```python
from build123d import *

# Parameters (mm, degrees)
SKETCH1_W           = 24
SKETCH1_H           = 24
BOSS_EXTRUDE1_DEPTH = 6
SKETCH2_W           = 24
SKETCH2_H           = 6
BOSS_EXTRUDE2_DEPTH = 30
SKETCH3_W           = 24
SKETCH3_H           = 6
BOSS_EXTRUDE3_DEPTH = 6
SKETCH4_W           = 24
SKETCH4_H           = 6
BOSS_EXTRUDE4_DEPTH = 6
SKETCH5_W           = 10
SKETCH5_H           = 6
BOSS_EXTRUDE5_DEPTH = 8
FILLET1_R           = 5
FILLET2_R           = 2
FILLET3_R           = 2
SKETCH6_W           = 10
SKETCH6_H           = 6
BOSS_EXTRUDE6_DEPTH = 8
FILLET4_R           = 5
FILLET5_R           = 2
SKETCH7_R           = 1.775
CUT_EXTRUDE1_DEPTH  = 42.568724431
CUT_EXTRUDE2_REACH  = 51.934
SKETCH8_R           = 1.75


with BuildPart() as part:
    # Sketch1 → Boss-Extrude1 (new body)
    with BuildSketch(Plane(origin=(0, 0, 0), x_dir=(1, 0, 0), z_dir=(0, 1, 0))):
        with Locations((1.896724894, -0.667948192)):
            Rectangle(SKETCH1_W, SKETCH1_H)
    extrude(amount=BOSS_EXTRUDE1_DEPTH)

    # Sketch2 → Boss-Extrude2 (add)
    with BuildSketch(Plane(origin=(0, 6, 0), x_dir=(1, 0, 0), z_dir=(0, 1, 0))):
        with Locations((1.896724894, -6.462948192)):
            Rectangle(SKETCH2_W, SKETCH2_H)
        with Locations((1.896724894, 5.127051808)):
            Rectangle(SKETCH2_W, SKETCH2_H)
    extrude(amount=BOSS_EXTRUDE2_DEPTH)

    # Sketch3 → Boss-Extrude3 (add)
    with BuildSketch(Plane.XY.offset(12.667948192)):
        with Locations((1.896724894, 3)):
            Rectangle(SKETCH3_W, SKETCH3_H)
    extrude(amount=BOSS_EXTRUDE3_DEPTH)

    # Sketch4 → Boss-Extrude4 (add)
    with BuildSketch(Plane(origin=(0, 0, -11.332051808), x_dir=(-1, 0, 0), z_dir=(0, 0, -1))):
        with Locations((-1.896724894, 3)):
            Rectangle(SKETCH4_W, SKETCH4_H)
    extrude(amount=BOSS_EXTRUDE4_DEPTH)

    # Sketch5 → Boss-Extrude5 (add)
    with BuildSketch(Plane(origin=(13.896724894, 0, 0), x_dir=(0, 0, -1), z_dir=(1, 0, 0))):
        with Locations((-0.667948192, 3)):
            Rectangle(SKETCH5_W, SKETCH5_H)
    extrude(amount=BOSS_EXTRUDE5_DEPTH)

    # Fillet1
    # the kernel refuses this fillet: 5 mm, written as the material it adds along each edge
    with BuildSketch(Plane(origin=(13.896724894, 0, -4.332051808), x_dir=(0, 0, -1), z_dir=(0, 1, 0)), Plane(origin=(13.896724894, 6, 5.667948192), x_dir=(0, 0, 1), z_dir=(0, -1, 0))) as fillet1_piece_1:
        with BuildLine():
            CenterArc((FILLET1_R, -FILLET1_R), FILLET1_R, 90, 90)
            Line((0, -FILLET1_R), (0, 0))
            Line((0, 0), (FILLET1_R, 0))
        make_face()
    extrude(amount=6)

    # Fillet2
    fillet2_edges = [part.edges().sort_by_distance(p)[0] for p in [
        (21.896724894, 3, -4.332051808),
        (21.896724894, 3, 5.667948192),
    ]]
    fillet(fillet2_edges, radius=FILLET2_R)

    # Fillet3
    fillet3_edges = [part.edges().sort_by_distance(p)[0] for p in [
        (-10.103275106, 3, 18.667948192),
        (13.896724894, 3, 18.667948192),
        (13.896724894, 3, -17.332051808),
        (-10.103275106, 3, -17.332051808),
    ]]
    fillet(fillet3_edges, radius=FILLET3_R)

    # Sketch6 → Boss-Extrude6 (add)
    with BuildSketch(Plane.ZY.offset(10.103275106)):
        with Locations((0.667948192, 3)):
            Rectangle(SKETCH6_W, SKETCH6_H)
    extrude(amount=BOSS_EXTRUDE6_DEPTH)

    # Fillet4
    # the kernel refuses this fillet: 5 mm, written as the material it adds along each edge
    with BuildSketch(Plane(origin=(-10.103275106, 6, -4.332051808), x_dir=(0, 0, -1), z_dir=(0, -1, 0)), Plane(origin=(-10.103275106, 0, 5.667948192), x_dir=(0, 0, 1), z_dir=(0, 1, 0))) as fillet4_piece_1:
        with BuildLine():
            CenterArc((FILLET4_R, -FILLET4_R), FILLET4_R, 90, 90)
            Line((0, -FILLET4_R), (0, 0))
            Line((0, 0), (FILLET4_R, 0))
        make_face()
    extrude(amount=6)

    # Fillet5
    fillet5_edges = [part.edges().sort_by_distance(p)[0] for p in [
        (-18.103275106, 3, -4.332051808),
        (-18.103275106, 3, 5.667948192),
    ]]
    fillet(fillet5_edges, radius=FILLET5_R)

    # Sketch7 → Cut-Extrude1 (cut, through all)
    with BuildSketch(Plane(origin=(0, 6, 0), x_dir=(1, 0, 0), z_dir=(0, 1, 0))):
        with Locations(Location((1.896724894, -13.667948192, 0), (0, 0, 270))):
            Circle(SKETCH7_R)
        with Locations(Location((-13.103275106, -0.667948192, 0), (0, 0, 270))):
            Circle(SKETCH7_R)
        with Locations(Location((1.896724894, 12.332051808, 0), (0, 0, 270))):
            Circle(SKETCH7_R)
        with Locations(Location((16.896724894, -0.667948192, 0), (0, 0, 270))):
            Circle(SKETCH7_R)
    extrude(amount=-CUT_EXTRUDE1_DEPTH, mode=Mode.SUBTRACT)

    # Cut-Extrude2: up to this face of the body (flat: up to its plane)
    cut_extrude2_end = Plane(part.part.faces().sort_by_distance((1.896724894, 21, -8.127051808))[0])
    # Sketch8 → Cut-Extrude2 (cut, up to the picked face)
    with BuildSketch(Plane.XY.offset(9.462948192), mode=Mode.PRIVATE) as cut_extrude2_sk1:
        with Locations((1.896724894, 15)):
            Circle(SKETCH8_R)
    cut_extrude2_tool1 = split(extrude(cut_extrude2_sk1.sketch, amount=-CUT_EXTRUDE2_REACH, mode=Mode.PRIVATE), bisect_by=cut_extrude2_end, keep=Keep.BOTH, mode=Mode.PRIVATE)
    # Sketch8 → Cut-Extrude2 (cut, up to the picked face)
    with BuildSketch(Plane.XY.offset(9.462948192), mode=Mode.PRIVATE) as cut_extrude2_sk2:
        with Locations((1.896724894, 25)):
            Circle(SKETCH8_R)
    cut_extrude2_tool2 = split(extrude(cut_extrude2_sk2.sketch, amount=-CUT_EXTRUDE2_REACH, mode=Mode.PRIVATE), bisect_by=cut_extrude2_end, keep=Keep.BOTH, mode=Mode.PRIVATE)
    add(cut_extrude2_tool1.solids().sort_by(Axis((1.896725, 15, 9.462948), (0, 0, -1)))[0], mode=Mode.SUBTRACT)
    add(cut_extrude2_tool2.solids().sort_by(Axis((1.896725, 25, 9.462948), (0, 0, -1)))[0], mode=Mode.SUBTRACT)


solid = part.part
```
Read the model definition and answer for the solid it produces. Units are mm, in the model's axes. A direction names the side the tool comes from. Give positions to 0.01 mm unless a question says otherwise; leave off trailing zeros. Loops run counter-clockwise (first coordinate to the right, second up) from the corner with the lowest first, then second, coordinate; pieces in that order, holes last.
Item 1: Each of these flat-tipped pins is pushed along its axis until it touches: pin 1 Ø7 at (x, y) = (6, 19.5) entering from +Z; pin 2 Ø1.8 at (y, z) = (14.5, -6.5) entering from +X; pin 3 Ø0.5 at (x, y) = (-15.5, 3.5) entering from -Z. Where does it stop, or does it pass through?
Item 2: The mould has two halves that part along Z. Classify faces 5 (the cylindrical face through (15.32, 2.96, -5.84)), 6 (the flat face through (-15.6, 3, 5.668)), 7 (the cylindrical face through (1.2, 3, -10.7)), 8 (the flat face through (2, 6, 0)): released by +Z, released by -Z, zero draft, split by the parting line, or undercut.
Item 3: The part is cut by section D-D (z = 7). Write down the section's boundary in (x, y).
Item 4: The part is cut by section C-C (z = 1.5). Write down the section's boundary in (x, y).
Item 5: For faces 1 (the flat face through (-15.6, 3, -4.332)), 2 (the flat face through (13.897, 3, 14)), 3 (the flat face through (2, 21, -8.127)), 4 (the flat face through (-10.103, 21, -5)), determine the directions among +Z, -Z, +X, -X, +Y, -Y from which every point of the face is accessible in a straight line to the end or side of a thin tool.
Item 6: The part is cut by section A-A (y = 15). Write down the section's boundary in (x, z), and give its area (3 significant figures).
Item 7: Find the intervals of material crossed by line 1 along Z through (x, y) = (9, 19.5); line 2 along X through (y, z) = (22, 5.5); line 3 along Y through (x, z) = (-6, -13), in increasing order.
Item 8: The part is cut by section B-B (x = -12.5). Write down the section's boundary in (y, z).
Taken from the geometry:
1. pin 1: stops at z = 9.46
1. pin 2: stops at x = 13.9
1. pin 3: stops at z = -4.33
2. face 5: released by -Z
2. face 6: released by +Z
2. face 7: undercut
2. face 8: undercut
3. outline: (-11.71, 0) - (15.5, 0) - (15.5, 6) - (13.9, 6) - (13.9, 36) - (-10.1, 36) - (-10.1, 6) - (-11.71, 6) - close; hole circle Ø3.5 at (1.9, 15); hole circle Ø3.5 at (1.9, 25)
4. outline: (-18.1, 0) - (-14.67, 0) - (-14.67, 6) - (-18.1, 6) - close; (-11.54, 0) - (15.33, 0) - (15.33, 6) - (-11.54, 6) - close; (18.46, 0) - (21.9, 0) - (21.9, 6) - (18.46, 6) - close
5. face 1: -Z, -X, +Y, -Y
5. face 2: +Z, +X, +Y, -Y
5. face 3: -Z, +X, -X, +Y
5. face 4: +Z, -Z, -X, +Y
6. outline: (-10.1, -8.13) - (0.15, -8.13) - (0.15, -2.13) - (-10.1, -2.13) - close; (-10.1, 3.46) - (0.15, 3.46) - (0.15, 9.46) - (-10.1, 9.46) - close; (3.65, -8.13) - (13.9, -8.13) - (13.9, -2.13) - (3.65, -2.13) - close; (3.65, 3.46) - (13.9, 3.46) - (13.9, 9.46) - (3.65, 9.46) - close
6. area: 246 mm2
7. line 1: z = -8.13 to -2.13, 3.46 to 9.46
7. line 2: x = -10.1 to 13.9
7. line 3: y = 0 to 6
8. outline: (0, -5.06) - (6, -5.06) - (6, -1) - (0, -1) - close; (0, 2.34) - (6, 2.34) - (6, 6.4) - (0, 6.4) - close
